from build123d import *

# Parameters (mm, degrees)
F0_R            = 279.4
F1_DEPTH        = 38.1
F2_R            = 279.4
F2_R_2          = 228.6
F3_DEPTH        = 6.35
F5_D            = 20.574
F6_R            = 101.6
F7_DEPTH        = 38.101
F8_R            = 158.75
F8_R_2          = 101.6
F9_DEPTH        = 6.35
F11_D           = 16.66748
F11_CSINK_D     = 30.1752
F11_CSINK_ANGLE = 82


with BuildPart() as f1:
    # F0 (on Front) → F1 (new body)
    with BuildSketch(Plane.XZ):
        Circle(F0_R)
    extrude(amount=F1_DEPTH)

    # F2 (on face) → F3 (cut)
    with BuildSketch(Plane.XZ.offset(38.1)):
        Circle(F2_R)
        Circle(F2_R_2, mode=Mode.SUBTRACT)
    extrude(amount=-F3_DEPTH, mode=Mode.SUBTRACT)

    # F5 (through all)
    with Locations(Plane.XZ.offset(31.75)):
        with Locations((179.6051224214, 179.6051224214), (254, 0), (179.6051224214, -179.6051224214), (0, -254), (-179.6051224214, -179.6051224214), (0, 254), (-179.6051224214, 179.6051224214), (-254, 0)):
            Hole(F5_D / 2)

    # F6 (on face) → F7 (cut, through all)
    with BuildSketch(Plane.XZ.offset(38.1)):
        Circle(F6_R)
    extrude(amount=-F7_DEPTH, mode=Mode.SUBTRACT)

    # F8 (on face) → F9 (cut)
    with BuildSketch(Plane(origin=(0, 0, 0), x_dir=(-1, 0, 0), z_dir=(0, 1, 0))):
        Circle(F8_R)
        Circle(F8_R_2, mode=Mode.SUBTRACT)
    extrude(amount=-F9_DEPTH, mode=Mode.SUBTRACT)

    # F11 (through all)
    with Locations(Plane.XZ.offset(38.1)):
        with Locations((139.7, 0), (98.7828173318, 98.7828173318), (0, 139.7), (-98.7828173318, 98.7828173318), (-139.7, 0), (-98.7828173318, -98.7828173318), (0, -139.7), (98.7828173318, -98.7828173318)):
            CounterSinkHole(F11_D / 2, F11_CSINK_D / 2, counter_sink_angle=F11_CSINK_ANGLE)


solid = f1.part
Check sheet for the modelled part. Datum: model origin and axes. Units: mm. Give positions to 0.01 mm unless a question says otherwise; leave off trailing zeros. Write each loop counter-clockwise with the first axis right and the second up, starting at its lowest first coordinate (ties: lowest second). Pieces come first, ordered by that corner, then holes. Notation, with made-up numbers: (-19.75, 54) -> (39.25, 54) arc R29 cw to (39.25, 83) -> close; hole circle Ø1 at (-2, 53.5). An arc over 180 degrees is marked (long way). One line per item, written item: value. Start each with the question number.
Item 1: Section check C-C on y = -21. State how many separate pieces and enclosed holes the cut face has, then the cut area to 3 significant figures.
Item 2: Draft check along Z on faces 1 (the flat face through (-43, -31.75, -226)), 2 (the conical face through (-3.997, -30.708, 132.016)). Enter one of: +Z half, -Z half, draft (parallel to the pull), parting line (faces both ways), or undercut.
Item 3: Gauge pin test, flat ends, axial feed: pin 1 (15 mm diameter, centred on x = 0, z = 139.7, fed in from +Y); pin 2 (12 mm diameter, centred on x = 106, z = 219.5, fed in from -Y); pin 3 (4 mm diameter, centred on y = -11.5, z = -202, fed in from +X); pin 4 (5 mm diameter, centred on y = -15.5, z = -20.5, fed in from -X). Record the tip position at first contact, or that the pin passes through.
Item 4: Section check A-A on x = -254. Record the cut outline in (y, z).
Item 5: Material ranges on probe 1 along Z at (x, y) = (186, -17); probe 2 along Y at (x, z) = (86, -123); probe 3 along X at (y, z) = (-32.5, -9), recorded low to high. Write a range as from..to.
Item 6: Section check B-B on z = -139.7. Record the cut outline in (x, y).
Results list:
1. separate pieces: 1
1. enclosed holes: 17
1. area: 208,000 mm²
2. face 1: draft
2. face 2: undercut
3. pin 1: through
3. pin 2: y = -31.75
3. pin 3: x = 195.1
3. pin 4: x = -278.82
4. outline: (-31.75, -116.4) -> (0, -116.4) -> (0, -10.29) -> (-31.75, -10.29) -> close; (-31.75, 10.29) -> (0, 10.29) -> (0, 116.4) -> (-31.75, 116.4) -> close
5. probe 1: -208.49..-187.66, -171.55..171.55, 187.66..208.49
5. probe 2: -38.1..-6.35
5. probe 3: -228.42..-144.54, -134.86..-101.2, 101.2..134.86, 144.54..228.42
6. outline: (-241.97, -31.75) -> (-180.95, -31.75) -> (-180.95, -38.1) -> (-15.09, -38.1) -> (-8.33, -30.33) -> (-8.33, -6.35) -> (-75.4, -6.35) -> (-75.4, 0) -> (-241.97, 0) -> close; (8.33, -30.33) -> (15.09, -38.1) -> (180.95, -38.1) -> (180.95, -31.75) -> (241.97, -31.75) -> (241.97, 0) -> (75.4, 0) -> (75.4, -6.35) -> (8.33, -6.35) -> close
